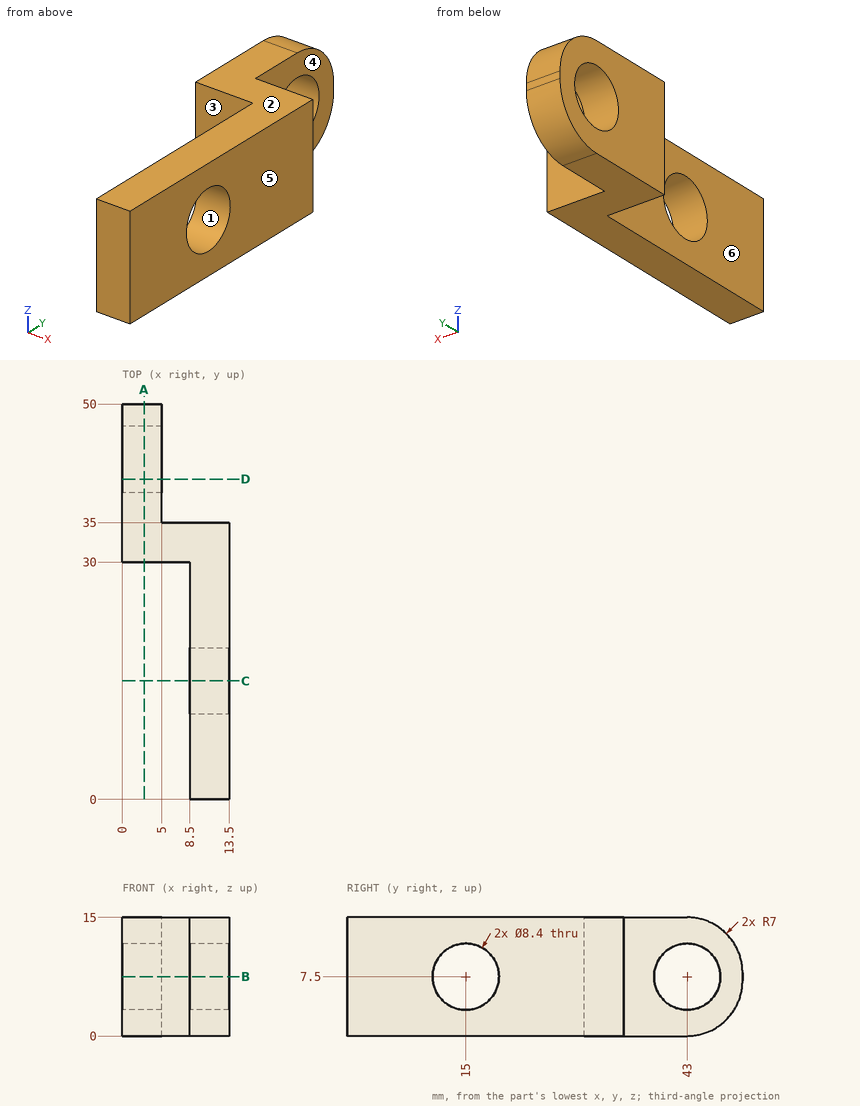
Source: three-view drawing plus pictorial views. Frame: mm from the lowest corner of the part. A direction names the side the tool comes from. Round coordinates to 2 decimals unless told otherwise and drop trailing zeros. Order: outer loops, then holes, each group sorted by start corner. A loop starts at its lowest first (then second) coordinate and runs counter-clockwise, first axis right, second up. Notation, with made-up numbers: (-30.75, 53.25) - (-26.75, 53.25) arc R33 ccw to (-26.75, 85.25) - close; hole circle Ø8 at (69.5, 59.25). An arc over 180 degrees is marked (long way). Answer in a Markdown table with one row per item.
Item 1: Mould query, pull axis Z, two halves, no side actions, for the marked faces 1, 2 and 3. Classes: released by +Z, released by -Z, zero draft, split by the parting line, or undercut.
Model answer:
| item | result |
|---|---|
| face 1 | undercut |
| face 2 | released by +Z |
| face 3 | zero draft |
Item 2: Reachability of the marked faces 4, 5 and 6 from +Z, -Z, +X, -X, +Y, -Y: full face, straight path, thin tool, end or side. Return the list, or none.
Model answer:
| item | result |
|---|---|
| face 4 | +Z, -Z, +X, +Y |
| face 5 | +Z, -Z, +X, +Y, -Y |
| face 6 | +Z, -Z, -X, -Y |
Item 3: Section query D-D (y = 40.5). Return the cut outline in (x, z), then the cut area to 3 significant figures.
Model answer:
| item | result |
|---|---|
| outline | (0, 0) - (5, 0) - (5, 4.13) - (0, 4.13) - close; (0, 10.87) - (5, 10.87) - (5, 15) - (0, 15) - close |
| area | 41.3 mm² |
Item 4: Section query C-C (y = 15). Return the cut outline in (x, z).
Model answer:
| item | result |
|---|---|
| outline | (8.5, 0) - (13.5, 0) - (13.5, 3.3) - (8.5, 3.3) - close; (8.5, 11.7) - (13.5, 11.7) - (13.5, 15) - (8.5, 15) - close |
Item 5: Section query A-A (x = 2.75). Return the cut outline in (y, z).
Model answer:
| item | result |
|---|---|
| outline | (30, 0) - (43, 0) arc R7 ccw to (50, 7) - (50, 8) arc R7 ccw to (43, 15) - (30, 15) - close; hole circle Ø8.4 at (43, 7.5) |
Item 6: Section query B-B (z = 7.5). Return the cut outline in (x, y), then the cut area to 4 significant figures.
Model answer:
| item | result |
|---|---|
| outline | (0, 30) - (8.5, 30) - (8.5, 19.2) - (13.5, 19.2) - (13.5, 35) - (5, 35) - (5, 38.8) - (0, 38.8) - close; (0, 47.2) - (5, 47.2) - (5, 50) - (0, 50) - close; (8.5, 0) - (13.5, 0) - (13.5, 10.8) - (8.5, 10.8) - close |
| area | 208.5 mm² |
Item 7: Pin query (flat end, axial travel): pin 1 (7.5 mm diameter, centred on y = 43, z = 7.5, fed in from -X); pin 2 (4 mm diameter, centred on x = 11, z = 11, fed in from +Y); pin 3 (7.5 mm diameter, centred on y = 42.5, z = 7.5, fed in from +X); pin 4 (4.5 mm diameter, centred on y = 16.5, z = 5.5, fed in from -X). Return the tip coordinate at first contact, or that it passes through.
Model answer:
| item | result |
|---|---|
| pin 1 | passes through |
| pin 2 | stops at y = 35 |
| pin 3 | stops at x = 5 |
| pin 4 | stops at x = 8.5 |
Item 8: Line query: line 1 (Z direction, x = 2.4, y = 43); line 2 (Y direction, x = 11.8, z = 7.5); line 3 (Y direction, x = 2.2, z = 7.5). Output: solid intervals per line, ascending.
Model answer:
| item | result |
|---|---|
| line 1 | z = 0 to 3.3, 11.7 to 15 |
| line 2 | y = 0 to 10.8, 19.2 to 35 |
| line 3 | y = 30 to 38.8, 47.2 to 50 |
